Autodesk Inventor part; units mm, degrees
ref_plane "Pracovní rovina1" through (9.25, -20, 0) normal (1, 0, 0) x (0, 0, -1)
ref_plane "Pracovní rovina2" through (27.25, -20, 0) normal (1, 0, 0) x (0, 0, -1)
ref_plane "YZ Plane" through (0, 0, 0) normal (1, 0, 0) x (0, 1, 0)
sketch "Náčrt1" plane through (0, 0, 0) normal (0, 0, 1) x (1, 0, 0)
  line L0 (0, 0) -> (54.5, 0)
  line L1 (54.5, 0) -> (54.5, -30.5)
  line L2 (0, -30.5) -> (0, 0)
  line L3 (0, -6.75) -> (-1, -6.75)
  line L4 (-1, -6.75) -> (-1, -20)
  line L5 (-1, -20) -> (0, -20)
  line L6 (54.5, -6.75) -> (55.5, -6.75)
  line L7 (55.5, -6.75) -> (55.5, -20)
  line L8 (55.5, -20) -> (54.5, -20)
  line L9 (54.5, -30.5) -> (43.25, -30.5)
  line L10 (43.25, -30.5) -> (43.25, -20.5)
  line L11 (43.25, -20.5) -> (11.25, -20.5)
  line L12 (11.25, -20.5) -> (11.25, -30.5)
  line L13 (11.25, -30.5) -> (0, -30.5)
  dimension "d0" = 54.5
  dimension "d1" = 30.5
  dimension "d3" = 13.25
  dimension "d4" = 1
  dimension "d5" = 1
  dimension "d6" = 13.25
  dimension "d17" = 10
  dimension "d18" = 11.25
  dimension "d41" = 10.5
  dimension "d42" = 10.5
extrude "Vysunutí1" add sketch "Náčrt1" along normal blind 2 contours L0 L1 L9 L10 L11 L12 L13 L2
extrude "Vysunutí2" add sketch "Náčrt1" along normal blind 2 and the other way blind 1 contours L2 L5 L4 L3 | L6 L7 L8 L1
chamfer "Zkosení1" distance 1 angle 45 2 edges at (-1, -13.375, 2) (55.5, -13.375, 2)
sketch "Náčrt2" plane through (0, 0, 2) normal (0, 0, 1) x (1, 0, 0)
  line L0 (43.25, -20.5) -> (43.25, -30.5)
  line L1 (54.5, -30.5) -> (54.5, -20)
  line L2 (43.25, -30.5) -> (54.5, -30.5)
  line L3 (49.375, -4.5) -> (54.5, -4.5) construction
  line L4 (54.5, -6.75) -> (54.5, 0)
  line L5 (5.125, -4.5) -> (0, -4.5) construction
  line L6 (0, 0) -> (0, -6.75)
  line L7 (54.5, 0) -> (0, 0)
  line L8 (0, -20) -> (0, -30.5)
  point P0 (49.875, -24.5)
  point P1 (4.625, -24.5)
  dimension "d20" = 6
  dimension "d28" = 44.25
  dimension "d31" = 6
  dimension "d50" = 4.625
  dimension "d51" = 4.5
  dimension "d52" = 4.625
hole "Díra2" at (49.875, -24.5, 2) at (49.375, -4.5, 2) at (5.125, -4.5, 2) at (4.625, -24.5, 2) direction (0, 0, -1) diameter 3.2 end through all
fillet "Zaoblení1" radius 5 2 edges at (0, 0, 1) (54.5, 0, 1)
ref_plane "Pracovní rovina1" through (9.25, -20, 0) normal (1, 0, 0) x (0, 0, -1)
sketch "Náčrt3" plane through (9.25, -20, 0) normal (1, 0, 0) x (0, 0, -1)
  line L0 (0, 0) -> (0, 13.25)
  line L1 (0, 1.5) -> (2.5, 1.5)
  line L2 (0, 11.75) -> (2.5, 11.75)
  line L3 (0, -10.5) -> (-2, -10.5)
  line L4 (0, 20) -> (-2, 20)
  arc A0 (2.5, 11.75) -> (2.5, 1.5) centre (6.5031, 6.625) ccw
  point P0 (0, 6.625)
  dimension "d43" = 10.25
  dimension "d44" = 2.5
  dimension "d45" = 12
  dimension "d47" = 6.5031
extrude "Vysunutí3" add sketch "Náčrt3" along normal blind 14.75
ref_plane "Pracovní rovina2" through (27.25, -20, 0) normal (1, 0, 0) x (0, 0, -1)
mirror "Zrcadlit1" about plane through (27.25, -20, 0) normal (1, 0, 0) of "Vysunutí3"
properties part number "objímka_motorů"
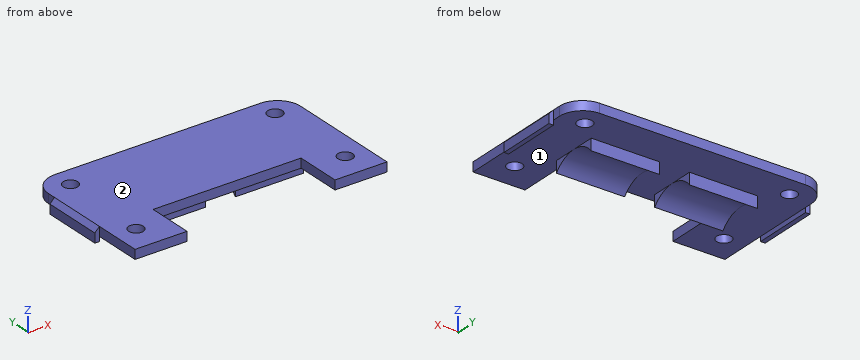
Verification items for the finished model (mm, model axes). Face numbers are marked on the shaded views. Coordinates: 2 decimals unless noted, no trailing zeros. Order: outer loops, then holes, each group sorted by start corner. A loop starts at its lowest first (then second) coordinate and runs counter-clockwise, first axis right, second up. Notation, with made-up numbers: M 23,20 L 28,20 A22 ccw 28,57 Z; hole C 13,68.25 d5. An arc over 180 degrees is marked long. One line per item, written item: value. Start each with the question number.
Item 1: Sectioned sample at C-C on z = -1.6. Record the cut outline in (x, y).
Item 2: Depth check by flat-ended pin: P1, Ø0.8, axis at x = -0.5, z = 1, coming from the -Y side; P2, Ø3, axis at x = 5.5, y = -27.5, coming from the -Z side; P3, Ø0.8, axis at x = -0.5, z = 1, coming from the +Y side. Enter the tip coordinate at first touch or a pass-through.
Item 3: Thickness scan on probe 1 along X at (y, z) = (-24.5, 1.3) (3 decimals); probe 2 along X at (y, z) = (-8.5, -1.15); probe 3 along X at (y, z) = (-4.5, 1.4) (3 decimals). Record the ranges inside material, lowest first.
Item 4: Sectioned sample at A-A on y = -24.5. Record the cut outline in (x, z) (3 decimals), then the cut area to 3 significant figures.
Item 5: Mould release check, pull along X, two halves, no side actions. Record for the marked faces 1 and 2: pulls with the +X half, pulls with the -X half, needs draft (parallel to the pull), parting line crosses it, or undercut.
Item 6: Sectioned sample at B-B on x = 21. Record the cut outline in (y, z) (3 decimals).
Item 7: Sectioned sample at D-D on y = -11.5. Record the cut outline in (x, z), then the cut area to 3 significant figures.
Calculated:
1. outline: M 9.25,-18.5 L 24,-18.5 L 24,-17.65 L 9.25,-17.65 Z; M 9.25,-9.1 L 24,-9.1 L 24,-8.25 L 9.25,-8.25 Z; M 30.5,-18.5 L 45.25,-18.5 L 45.25,-17.65 L 30.5,-17.65 Z; M 30.5,-9.1 L 45.25,-9.1 L 45.25,-8.25 L 30.5,-8.25 Z
2. P1: y = -20
2. P2: z = 0
2. P3: y = -6.75
3. probe 1: 0 to 3.025, 6.225 to 11.25, 43.25 to 48.275, 51.475 to 54.5
3. probe 2: 9.25 to 24, 30.5 to 45.25
3. probe 3: 0.025 to 3.525, 6.725 to 47.775, 50.975 to 54.475
4. outline: M 0,0 L 3.025,0 L 3.025,2 L 0,2 Z; M 6.225,0 L 11.25,0 L 11.25,2 L 6.225,2 Z; M 43.25,0 L 48.275,0 L 48.275,2 L 43.25,2 Z; M 51.475,0 L 54.5,0 L 54.5,2 L 51.475,2 Z
4. area: 32.2 mm^2
5. face 1: undercut
5. face 2: needs draft
6. outline: M -20.5,0 L -18.5,0 L -18.5,-2.5 A6.503 cw -8.25,-2.5 L -8.25,0 L 0,0 L 0,2 L -20.5,2 Z
7. outline: M -1,-1 L 0,-1 L 0,0 L 9.25,0 L 9.25,-0.28 L 24,-0.28 L 24,0 L 30.5,0 L 30.5,-0.28 L 45.25,-0.28 L 45.25,0 L 54.5,0 L 54.5,-1 L 55.5,-1 L 55.5,1 L 54.5,2 L 0,2 L -1,1 Z
7. area: 122 mm^2
